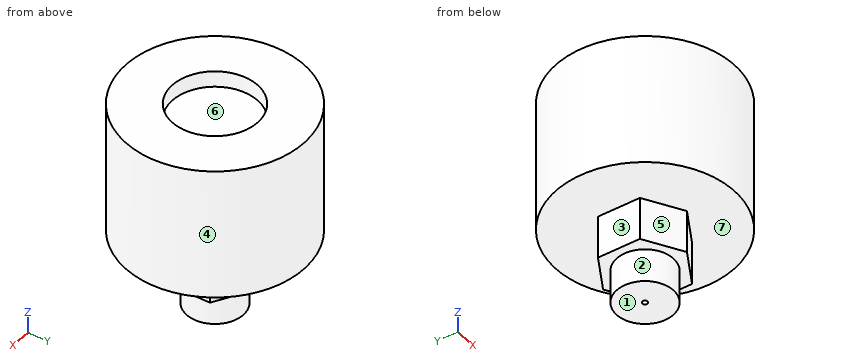
from build123d import *

# Parameters (mm, degrees)
BOSS_EXTRUDE1_DEPTH      = 1
BOSS_EXTRUDE1_DEPTH_BACK = 0.5
SKETCH3_R                = 8.35
SKETCH3_R_2              = 4
SKETCH4_R                = 8.35
BOSS_EXTRUDE2_DEPTH      = 10.8
BOSS_EXTRUDE4_DEPTH      = 4
SKETCH6_R                = 2.65
BOSS_EXTRUDE5_DEPTH      = 3.1
SKETCH7_R                = 0.244312337
CUT_EXTRUDE1_DEPTH       = 2


with BuildPart() as part:
    # Sketch3 → Boss-Extrude1 (new, two sides: drawn at the far end of the back side and taken through both)
    with BuildSketch(Plane.XY.offset(-BOSS_EXTRUDE1_DEPTH_BACK)):
        Circle(SKETCH3_R)
        Circle(SKETCH3_R_2, mode=Mode.SUBTRACT)
    extrude(amount=BOSS_EXTRUDE1_DEPTH + BOSS_EXTRUDE1_DEPTH_BACK)

    # Sketch4 → Boss-Extrude2 (add)
    with BuildSketch(Plane(origin=(0, 0, -0.5), x_dir=(-1, 0, 0), z_dir=(0, 0, -1))):
        with Locations(Location((0, 0, 0), (0, 0, 180))):
            Circle(SKETCH4_R)
    extrude(amount=BOSS_EXTRUDE2_DEPTH)

    # Sketch5 → Boss-Extrude4 (add)
    with BuildSketch(Plane(origin=(0, 0, -11.3), x_dir=(-1, 0, 0), z_dir=(0, 0, -1))):
        Polygon((0, 3.95), (-3.420800345, 1.975), (-3.420800345, -1.975), (0, -3.95), (3.420800345, -1.975), (3.420800345, 1.975), align=None)
    extrude(amount=BOSS_EXTRUDE4_DEPTH)

    # Sketch6 → Boss-Extrude5 (add)
    with BuildSketch(Plane(origin=(0, 0, -15.3), x_dir=(-1, 0, 0), z_dir=(0, 0, -1))):
        with Locations(Location((0, 0, 0), (0, 0, 180))):
            Circle(SKETCH6_R)
    extrude(amount=BOSS_EXTRUDE5_DEPTH)

    # Sketch7 → Cut-Extrude1 (cut)
    with BuildSketch(Plane(origin=(0, 0, -18.4), x_dir=(-1, 0, 0), z_dir=(0, 0, -1))):
        Circle(SKETCH7_R)
    extrude(amount=-CUT_EXTRUDE1_DEPTH, mode=Mode.SUBTRACT)


solid = part.part
Here's how the part is built. I have some questions about the finished solid (model axes, mm). Face numbers are marked on the shaded views. A direction names the side the tool comes from. Coordinates: 2 decimals unless noted, no trailing zeros. Order: outer loops, then holes, each group sorted by start corner. A loop starts at its lowest first (then second) coordinate and runs counter-clockwise, first axis right, second up. Notation, with made-up numbers: M 13.25,35.25 L 59.25,35.25 A26 ccw 59.25,59.25 Z; hole C 69.25,-17.75 d4. An arc over 180 degrees is marked long. Answer as CSV lines item,"result". Start each with the question number.
1. On a 3-axis mill with a long thin cutter (end or side, diameter ignored), from which of +Z, -Z, +X, -X, +Y, -Y can I reach the whole of each face in a straight line? I mean the marked faces 1, 2 and 3. Say none if no direction works.
2. I need wall thicknesses on line 1 (Y direction, x = 0, z = -17.45); line 2 (Y direction, x = 0, z = 0.25); line 3 (Z direction, x = 6, y = 4). Which ranges of each line are inside material? Lowest first, please. Write a range as [from, to].
3. We'd pull the mould along X, two halves only. Please class the marked faces 4, 5, 6 and 7: released by +X, released by -X, zero draft, split by the parting line, or undercut.
4. For pin 1 (2 mm diameter, centred on x = 6, y = -3.5, fed in from -Z); pin 2 (10 mm diameter, centred on x = -6, y = 0.5, fed in from -Z); pin 3 (3 mm diameter, centred on x = 6.5, z = -11, fed in from +Y); pin 4 (4.5 mm diameter, centred on y = 0, z = -14, fed in from -X), each with a flat end and sliding along its axis, tell me the tip position at first contact or that it passes through.
5. I want a section at D-D, the plane y = 1.5. Write out the boundary of the cut face in (x, z), and give its area (3 significant figures).
6. I want a section at C-C, the plane x = -5. Write out the boundary of the cut face in (y, z).
7. I want a section at A-A, the plane y = 3.5. Write out the boundary of the cut face in (x, z).
8. I want a section at B-B, the plane z = -11.75. Write out the boundary of the cut face in (x, y) (3 decimals), and give its area (3 significant figures).
Recorded:
1,face 1,"-Z, +X, -X, +Y, -Y"
1,face 2,"-Z"
1,face 3,"-Z, -X, +Y, -Y"
2,line 1,"y = [-2.65, -0.24], [0.24, 2.65]"
2,line 2,"y = [-8.35, -4], [4, 8.35]"
2,line 3,"z = [-11.3, 1]"
3,face 4,"split by the parting line"
3,face 5,"released by -X"
3,face 6,"undercut"
3,face 7,"zero draft"
4,pin 1,"stops at z = -11.3"
4,pin 2,"stops at z = -18.4"
4,pin 3,"stops at y = 6.69"
4,pin 4,"stops at x = -3.42"
5,outline,"M -8.21,-11.3 L -3.42,-11.3 L -3.42,-15.3 L -2.18,-15.3 L -2.18,-18.4 L 2.18,-18.4 L 2.18,-15.3 L 3.42,-15.3 L 3.42,-11.3 L 8.21,-11.3 L 8.21,1 L 3.71,1 L 3.71,-0.5 L -3.71,-0.5 L -3.71,1 L -8.21,1 Z"
5,area,"232 mm2"
6,outline,"M -6.69,-11.3 L 6.69,-11.3 L 6.69,1 L -6.69,1 Z"
7,outline,"M -7.58,-11.3 L -0.78,-11.3 L -0.78,-15.3 L 0.78,-15.3 L 0.78,-11.3 L 7.58,-11.3 L 7.58,1 L 1.94,1 L 1.94,-0.5 L -1.94,-0.5 L -1.94,1 L -7.58,1 Z"
8,outline,"M -3.421,-1.975 L 0,-3.95 L 3.421,-1.975 L 3.421,1.975 L 0,3.95 L -3.421,1.975 Z"
8,area,"40.5 mm2"
